CAD build for the part. Positions are in the model's coordinates, mm. Give positions to 0.01 mm unless a question says otherwise; leave off trailing zeros. Loops run counter-clockwise (first coordinate to the right, second up) from the corner with the lowest first, then second, coordinate; pieces in that order, holes last. Notation, with made-up numbers: (69.25, 16) -> (113.25, 16) arc R13 ccw to (113.25, 22) -> close; hole circle Ø7 at (10, 64.5). An arc over 180 degrees is marked (long way). Use one line per item in the form item = value.
```python
from build123d import *

# Parameters (mm, degrees)
F0_W     = 14.6
F0_H     = 7.3
F1_DEPTH = 10
F2_R     = 0.25
F3_DEPTH = 3.2


with BuildPart() as f1:
    # F0 (on Top) → F1 (new body)
    with BuildSketch(Plane.XY):
        with Locations((7.3, 3.65)):
            Rectangle(F0_W, F0_H)
    extrude(amount=F1_DEPTH)

    # F2 (on face) → F3 (join)
    with BuildSketch(Plane.XY.offset(10)):
        with Locations((2.196679, 5.826643)):
            Circle(F2_R)
        with Locations((2.196679, 1.473357)):
            Circle(F2_R)
        with Locations((6.117353, 1.473357)):
            Circle(F2_R)
        with Locations((6.117353, 5.826643)):
            Circle(F2_R)
        with Locations((8.857069, 5.826643)):
            Circle(F2_R)
        with Locations((11.597946, 5.826643)):
            Circle(F2_R)
        with Locations((11.597946, 1.473357)):
            Circle(F2_R)
        with Locations((8.857069, 1.473357)):
            Circle(F2_R)
    extrude(amount=F3_DEPTH)


solid = f1.part
```
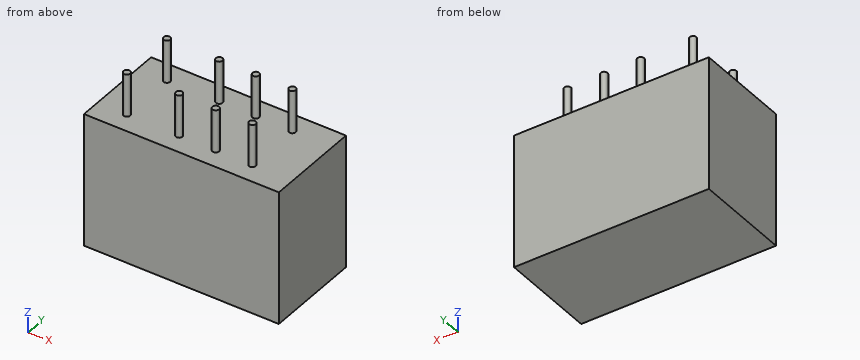
1. Cut at B-B, the plane y = 0.5. Write the cut outline in (x, z).
Result sheet:
outline = (0, 0) -> (14.6, 0) -> (14.6, 10) -> (0, 10) -> close
2. Cut at A-A, the plane z = 11.25. Write the cut outline in (x, y).
Result sheet:
outline = circle Ø0.5 at (2.2, 1.47); circle Ø0.5 at (2.2, 5.83); circle Ø0.5 at (6.12, 1.47); circle Ø0.5 at (6.12, 5.83); circle Ø0.5 at (8.86, 1.47); circle Ø0.5 at (8.86, 5.83); circle Ø0.5 at (11.6, 1.47); circle Ø0.5 at (11.6, 5.83)
3. Cut at C-C, the plane x = 5. Write the cut outline in (y, z).
Result sheet:
outline = (0, 0) -> (7.3, 0) -> (7.3, 10) -> (0, 10) -> close
4. Drill centre lines: line 1 (Z direction, x = 7.5, y = 3); line 2 (Y direction, x = 11.5, z = 11.25). Where is each one in solid material? Low to high.
Result sheet:
line_1 = 0 to 10
line_2 = 1.24 to 1.7, 5.6 to 6.06
